```python
from build123d import *

# Parameters (mm, degrees)
BOSS_EXTRUDE1_DEPTH = 5
CUT_EXTRUDE1_DEPTH  = 6
CAVITY1_DEPTH       = 5


# Read off the part's stored shape, not the designer's step: Cavity1
with BuildPart() as part:
    # Sketch3 → Boss-Extrude1 (new body)
    with BuildSketch(Plane(origin=(0, 0, 0), x_dir=(0, 0, -1), z_dir=(1, 0, 0))):
        with BuildLine():
            ThreePointArc((0, 60), (-13.5, 46.5), (0, 33))
            ThreePointArc((0, 33), (48.489461609, -8.147530745), (10.41889066, -59.088465181))
            ThreePointArc((10.41889066, -59.088465181), (5.229344565, -59.771681886), (0, -60))
            ThreePointArc((0, -60), (13.5, -46.5), (0, -33))
            ThreePointArc((0, -33), (-48.489461609, 8.147530745), (-10.41889066, 59.088465181))
            ThreePointArc((-10.41889066, 59.088465181), (-5.229344565, 59.771681886), (0, 60))
        make_face()
    extrude(amount=BOSS_EXTRUDE1_DEPTH)

    # Sketch5 → Cut-Extrude1 (cut)
    with BuildSketch(Plane(origin=(0, 0, 0), x_dir=(0, 0, -1), z_dir=(1, 0, 0))):
        Polygon((-5, 59.039936204), (0, 63.23543436), (4.195498156, 58.23543436), (-0.804501844, 54.039936204), align=None)
        Polygon((5, -59.039936204), (0, -63.23543436), (-4.195498156, -58.23543436), (0.804501844, -54.039936204), align=None)
    extrude(amount=CUT_EXTRUDE1_DEPTH, mode=Mode.SUBTRACT)

    # Cavity1 outline → Cavity1 (cut)
    with BuildSketch(Plane.YZ):
        Polygon((-18.108015498, 4.108286468), (-12.544428042, -13.539583883), (5.520869734, -17.545310986), (18.022580053, -3.903167737), (12.458992597, 13.744702615), (-5.606305179, 17.750429717), align=None)
    extrude(amount=CAVITY1_DEPTH, mode=Mode.SUBTRACT)


solid = part.part
```
Here's how the part is built. I have some questions about the finished solid (model axes, mm). A direction names the side the tool comes from. Round coordinates to 2 decimals unless told otherwise and drop trailing zeros. Order: outer loops, then holes, each group sorted by start corner. A loop starts at its lowest first (then second) coordinate and runs counter-clockwise, first axis right, second up. Notation, with made-up numbers: M 55,85.5 L 101,85.5 A24 ccw 101,96.5 Z; hole C 57.25,50.25 d7. An arc over 180 degrees is marked long. Answer as CSV lines item,"result".
Item 1: Imagine slicing it at D-D on z = 21.5. List the corners of the cut face in (x, y) for me, and give its area (3 significant figures).
From the geometry:
outline,"M 0,-28.93 L 5,-28.93 L 5,55.66 L 0,55.66 Z"
area,"423 mm2"
Item 2: Imagine slicing it at C-C on z = 9. List the corners of the cut face in (x, y) for me.
From the geometry:
outline,"M 0,-32.58 L 5,-32.58 L 5,-13.63 L 0,-13.63 Z; M 0,13.95 L 5,13.95 L 5,36.44 L 0,36.44 Z; M 0,56.56 L 5,56.56 L 5,59.32 L 0,59.32 Z"
Item 3: Imagine slicing it at A-A on x = 2.2. List the corners of the cut face in (y, z) for me.
From the geometry:
outline,"M -59.87,-4.02 A60 ccw -59.09,-10.42 A46.43 ccw 33,0 A13.5 cw 59.04,5 L 59.87,4.02 A60 ccw 59.09,10.42 A46.43 ccw -33,0 A13.5 cw -59.04,-5 Z; hole M -18.11,4.11 L -12.54,-13.54 L 5.52,-17.55 L 18.02,-3.9 L 12.46,13.74 L -5.61,17.75 Z"
Item 4: Imagine slicing it at B-B on y = 8.5. List the corners of the cut face in (x, z) for me, and give its area (3 significant figures).
From the geometry:
outline,"M 0,-43.31 L 5,-43.31 L 5,-14.29 L 0,-14.29 Z; M 0,14.62 L 5,14.62 L 5,48.53 L 0,48.53 Z"
area,"315 mm2"
Item 5: For pin 1 (1.5 mm diameter, centred on x = 2, y = 28.5, fed in from -Z); pin 2 (2 mm diameter, centred on x = 2.5, y = 28.5, fed in from +Z); pin 3 (1.5 mm diameter, centred on x = 3, z = 34, fed in from +Y), each with a flat end and sliding along its axis, tell me the tip position at first contact or that it passes through.
From the geometry:
pin 1,"z = -23.92"
pin 2,"z = 46.58"
pin 3,"y = 48.02"
Item 6: We'd pull the mould along Z, two halves only. Please class faces 3 (the flat face through (2.465, -3.638, -15.514)), 4 (the cylindrical face through (2.465, -59.558, -7.273)), 5 (the flat face through (5, 14, -12)), 6 (the flat face through (2.46, 15.28, 4.8)): +Z half, -Z half, draft (parallel to the pull), parting line (faces both ways), or undercut.
From the geometry:
face 3,"undercut"
face 4,"-Z half"
face 5,"draft"
face 6,"undercut"
Item 7: Please list where these lines run through material, in increasing order: L1, parallel to Y at x = 3.05, z = 6; L2, parallel to Y at x = 3.95, z = 11; L3, parallel to Y at x = 2.1, z = 26.5. Write a range as [from, to].
From the geometry:
L1,"[-32.92, -16.37], [14.9, 34.41], [58.59, 59.7]"
L2,"[-32.25, -11.79], [13.32, 38.67], [54.33, 58.98]"
L3,"[-26.29, 53.02]"
Item 8: Which directions (+Z, -Z, +X, -X, +Y, -Y) give clear straight access to the entire face, cutting with the end or side of a thin tool? Please do faces 1 (the cylindrical face through (2.465, 59.558, 7.273)), 2 (the flat face through (2.465, -11.77, 11.025)).
From the geometry:
face 1,"+Z, +X, -X, +Y"
face 2,"+X, -X"
